from build123d import *

# Parameters (mm, degrees)
F1_DEPTH      = 17.9
F0_W          = 2.9
F0_H          = 16.5
F0_H_2        = 1.5
F2_DEPTH      = 18
F2_DEPTH_BACK = 1.5
F4_D          = 3.3


# Not quite as in the source:
# - a feature names something its author has since deleted; it is built from what else it names


with BuildPart() as f1:
    # F0 (on Right) → F1 (new body)
    with BuildSketch(Plane.YZ):
        Polygon((3.4158524887, 16.5), (2.3158524887, 16.5), (2.3158524887, 0), (3.4158524887, 0), (3.4158524887, 7.4381744285), align=None)
        with BuildLine():
            ThreePointArc((7.9540269172, 2.9), (4.7450530046, 4.2292005159), (3.4158524887, 7.4381744285))
            Line((3.4158524887, 7.4381744285), (3.4158524887, 0))
            Line((3.4158524887, 0), (9.4158524887, 0))
            Line((9.4158524887, 0), (12.5158524887, 0))
            Line((12.5158524887, 0), (22.0158524887, 0))
            Line((22.0158524887, 0), (25.1158524887, 0))
            Line((25.1158524887, 0), (28.1158524887, 0))
            Line((28.1158524887, 0), (28.1158524887, 2.9))
            Line((28.1158524887, 2.9), (25.1158524887, 2.9))
            Line((25.1158524887, 2.9), (22.0158524887, 2.9))
            Line((22.0158524887, 2.9), (12.5158524887, 2.9))
            Line((12.5158524887, 2.9), (9.4158524887, 2.9))
            Line((9.4158524887, 2.9), (7.9540269172, 2.9))
        make_face()
    extrude(amount=F1_DEPTH)

    # F0 (on Right) → F2 (join, two sides)
    with BuildSketch(Plane.YZ) as f2_sk:
        with Locations((0.8658524887, 8.25)):
            Rectangle(F0_W, F0_H)
        Polygon((-0.5841475113, 18.1), (-0.5841475113, 16.5), (2.3158524887, 16.5), (2.3158524887, 18.1), (3.4158524887, 18.1), (1.4158524887, 38.1), (-0.5841475113, 38.1), align=None)
        with Locations((0.8658524887, -0.75)):
            Rectangle(F0_W, F0_H_2)
    extrude(amount=F2_DEPTH)
    extrude(f2_sk.sketch, amount=-F2_DEPTH_BACK)

    # F4 (through all)
    with Locations(Plane(origin=(0, 0, 0), x_dir=(1, 0, 0), z_dir=(0, 0, -1))):
        with Locations((8.95, -9.3158524887), (8.95, -18.8158524887)):
            Hole(F4_D / 2)


solid = f1.part
Input: part model. Units: mm. Frame: model coordinates. A direction names the side the tool comes from. Coordinates: 2 decimals unless noted, no trailing zeros. Loops run counter-clockwise (first coordinate to the right, second up) from the corner with the lowest first, then second, coordinate; pieces in that order, holes last. Notation, with made-up numbers: (-6.75, -19.5) -> (15.25, -19.5) arc R30 cw to (15.25, 13.5) -> close; hole circle Ø2 at (39, 28.25). An arc over 180 degrees is marked (long way). Write each question's results on one line, items separated by ' | '. Start each with the question number.
Q1. Section C-C, the plane x = 12.25. Return the cut outline in (y, z), plus the area to 3 significant figures.
Q2. Reachability of faces 1 (the flat face through (9, 15, 0)), 2 (the flat face through (0, 13, 2)), 3 (the flat face through (9, 3.416, 12)) from +Z, -Z, +X, -X, +Y, -Y: full face, straight path, thin tool, end or side. Return the list, or none.
Q3. Section A-A, the plane x = 8.95. Return the cut outline in (y, z).
Q4. Pull-direction query (Z, two-part tool) for faces 4 (the flat face through (8, 3, 18.1)), 5 (the flat face through (-0.4, 2.316, 8.3)), 6 (the cylindrical face through (8.825, 4.781, 4.194)), 7 (the flat face through (9, 28.116, 1)); classes: released by +Z, released by -Z, zero draft, split by the parting line, or undercut.
Q5. Ray query, line 1 (Y direction, x = 8.95, z = 1.1); line 2 (Z direction, x = 10.75, y = 18); line 3 (Y direction, x = 2.5, z = 12). Return the intervals inside material, ascending. Write a range as from..to.
Q6. Section B-B, the plane z = 9. Return the cut outline in (x, y), plus the area to 3 significant figures.
Q7. Section D-D, the plane y = 15.5. Return the cut outline in (x, z), plus the area to 3 significant figures.
Q8. Pin query (flat end, axial travel): pin 1 (1.2 mm diameter, centred on x = 11, y = 3, fed in from -Z); pin 2 (5 mm diameter, centred on x = 7.5, z = 31.5, fed in from +Y); pin 3 (5.5 mm diameter, centred on x = 8.95, y = 9.32, fed in from +Z). Return the tip coordinate at first contact, or that it passes through.
Found:
1) outline: (-0.58, -1.5) -> (2.32, -1.5) -> (2.32, 0) -> (28.12, 0) -> (28.12, 2.9) -> (7.95, 2.9) arc R4.54 cw to (3.42, 7.44) -> (3.42, 16.5) -> (2.32, 16.5) -> (2.32, 18.1) -> (3.42, 18.1) -> (1.42, 38.1) -> (-0.58, 38.1) -> close | area: 211 mm2
2) face 1: -Z, +X, -X, +Y | face 2: -Z, -X, +Y | face 3: +Z, +X, -X, +Y
3) outline: (-0.58, -1.5) -> (2.32, -1.5) -> (2.32, 0) -> (7.67, 0) -> (7.67, 2.91) arc R4.54 cw to (3.42, 7.44) -> (3.42, 16.5) -> (2.32, 16.5) -> (2.32, 18.1) -> (3.42, 18.1) -> (1.42, 38.1) -> (-0.58, 38.1) -> close; (10.97, 0) -> (17.17, 0) -> (17.17, 2.9) -> (10.97, 2.9) -> close; (20.47, 0) -> (28.12, 0) -> (28.12, 2.9) -> (20.47, 2.9) -> close
4) face 4: undercut | face 5: undercut | face 6: released by +Z | face 7: zero draft
5) line 1: -0.58..7.67, 10.97..17.17, 20.47..28.12 | line 2: 0..2.9 | line 3: -0.58..3.42
6) outline: (-1.5, -0.58) -> (18, -0.58) -> (18, 2.32) -> (17.9, 2.32) -> (17.9, 3.42) -> (0, 3.42) -> (0, 2.32) -> (-1.5, 2.32) -> close | area: 76.2 mm2
7) outline: (0, 0) -> (17.9, 0) -> (17.9, 2.9) -> (0, 2.9) -> close | area: 51.9 mm2
8) pin 1: z = 0 | pin 2: y = 2.33 | pin 3: z = 3.12
